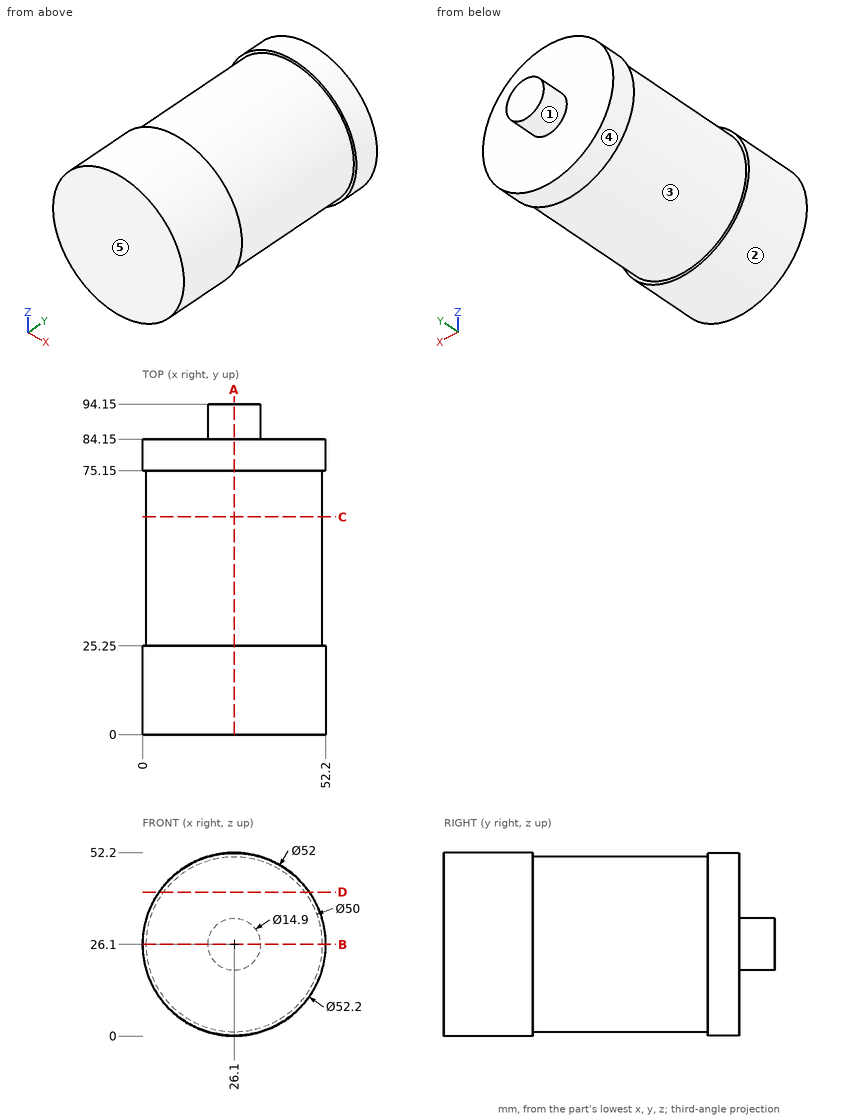
Can you work these out from the drawing? Everything is in mm from the part's minimum corner. A direction names the side the tool comes from. Round coordinates to 2 decimals unless told otherwise and drop trailing zeros. Loops run counter-clockwise (first coordinate to the right, second up) from the corner with the lowest first, then second, coordinate; pieces in that order, holes last. Notation, with made-up numbers: (-27.75, 70) -> (25.25, 70) arc R20 ccw to (25.25, 78) -> close; hole circle Ø10 at (29, 55). An arc over 180 degrees is marked (long way). Put each result on its own line as item: value.
Q1. Thinking about a two-plate mould opening in Y: for the marked faces 3, 4 and 5, which applies, pulls with the +Y half, pulls with the -Y half, needs draft (parallel to the pull), parting line crosses it, or undercut?
Checks:
face 3: undercut
face 4: needs draft
face 5: pulls with the -Y half
Q2. Please list where these lines run through material, in increasing order: line 1 (Y direction, x = 15.5, z = 49.5); line 2 (Y direction, x = 39.5, z = 14.5); line 3 (Z direction, x = 3, y = 56.5). Write a range as from..to.
Checks:
line 1: 0..25.25, 75.15..84.15
line 2: 0..84.15
line 3: 16.54..35.66
Q3. I want a section at A-A on x = 26.1. Write out the boundary of the cut face in (y, z).
Checks:
outline: (0, 0) -> (25.25, 0) -> (25.25, 1.1) -> (75.15, 1.1) -> (75.15, 0.1) -> (84.15, 0.1) -> (84.15, 18.65) -> (94.15, 18.65) -> (94.15, 33.55) -> (84.15, 33.55) -> (84.15, 52.1) -> (75.15, 52.1) -> (75.15, 51.1) -> (25.25, 51.1) -> (25.25, 52.2) -> (0, 52.2) -> close
Q4. For pin 1 Ø8 at (x, y) = (9.5, 42) entering from +Z; pin 2 Ø12 at (y, z) = (57.5, 19) entering from +X; pin 3 Ø4 at (x, y) = (43.5, 63.5) entering from -Z; pin 4 Ø8 at (x, z) = (12, 29.5) entering from -Y, each with a flat end and sliding along its axis, tell me the tip position at first contact or that it passes through.
Checks:
pin 1: z = 47.69
pin 2: x = 51.08
pin 3: z = 6.41
pin 4: y = 0
Q5. I want a section at C-C on y = 62. Write out the boundary of the cut face in (x, z).
Checks:
outline: circle Ø50 at (26.1, 26.1)
Q6. Which directions (+Z, -Z, +X, -X, +Y, -Y) give clear straight access to the entire face, cutting with the end or side of a thin tool? Please do the marked faces 1 and 2.
Checks:
face 1: +Y
face 2: +Y, -Y
Q7. I want a section at B-B on z = 26.1. Write out the boundary of the cut face in (x, y), and give its area (3 significant figures).
Checks:
outline: (0, 0) -> (52.2, 0) -> (52.2, 25.25) -> (51.1, 25.25) -> (51.1, 75.15) -> (52.1, 75.15) -> (52.1, 84.15) -> (33.55, 84.15) -> (33.55, 94.15) -> (18.65, 94.15) -> (18.65, 84.15) -> (0.1, 84.15) -> (0.1, 75.15) -> (1.1, 75.15) -> (1.1, 25.25) -> (0, 25.25) -> close
area: 4,430 mm2
Q8. I want a section at D-D on z = 41. Write out the boundary of the cut face in (x, y), and give its area (3 significant figures).
Checks:
outline: (4.67, 0) -> (47.53, 0) -> (47.53, 25.25) -> (46.17, 25.25) -> (46.17, 75.15) -> (47.41, 75.15) -> (47.41, 84.15) -> (4.79, 84.15) -> (4.79, 75.15) -> (6.03, 75.15) -> (6.03, 25.25) -> (4.67, 25.25) -> close
area: 3,470 mm2
